Autodesk Inventor part; units mm, degrees
ref_plane "YZ Plane" through (0, 0, 0) normal (1, 0, 0) x (0, 1, 0)
ref_plane "XZ Plane" through (0, 0, 0) normal (0, 1, 0) x (-1, 0, 0)
ref_plane "XY Plane" through (0, 0, 0) normal (0, 0, 1) x (1, 0, 0)
sketch "Sketch1" plane through (0, 0, 0) normal (0, 1, 0) x (-1, 0, 0)
  line L0 (2, -96) -> (-2, -96)
  line L1 (-2, -96) -> (-2, 96)
  line L2 (-2, 96) -> (2, 96)
  line L3 (2, 96) -> (2, -96)
  line L4 (2, -96) -> (-2, 96) construction
  line L5 (-2, -96) -> (2, 96) construction
  circle A0 centre (0, 94) radius 0.85
  circle A1 centre (0, -94) radius 0.85
  circle A2 centre (0, 0) radius 0.85
  circle A3 centre (0, 48) radius 0.85
  circle A4 centre (0, -48) radius 0.85
  point P0 (0, 0)
  dimension "d0" = 192
  dimension "d1" = 4
  dimension "d2" = 1.7
  dimension "d3" = 2
  dimension "d4" = 2
  dimension "d5" = 1.7
  dimension "d6" = 2
  dimension "d7" = 2
  dimension "d8" = 1.7
  dimension "d9" = 96
  dimension "d10" = 2
  dimension "d11" = 1.7
  dimension "d12" = 2
  dimension "d13" = 48
  dimension "d14" = 1.7
  dimension "d15" = 2
  dimension "d16" = 48
extrude "MainBody" add sketch "Sketch1" along normal blind 70
sketch "Sketch2" plane through (0, 70, 0) normal (0, 1, 0) x (1, 0, 0)
  circle A0 centre (0, 0) radius 0.85
extrude "MiddlePole" add sketch "Sketch2" along normal blind 3 and the other way blind 70
sketch "Sketch3" plane through (0, 70, 0) normal (0, 1, 0) x (1, 0, 0)
  circle A0 centre (0, -48) radius 0.85
  point P0 (0, 0)
extrude "MiddleLeftPole" add sketch "Sketch3" along normal blind 3 and the other way blind 70
sketch "Sketch4" plane through (0, 70, 0) normal (0, 1, 0) x (1, 0, 0)
  circle A0 centre (0, -94) radius 0.85
  point P0 (0, 0)
extrude "LeftMostPole" add sketch "Sketch4" along normal blind 3 and the other way blind 70
sketch "Sketch5" plane through (0, 70, 0) normal (0, 1, 0) x (1, 0, 0)
  circle A0 centre (0, 48) radius 0.85
  point P0 (0, 0)
extrude "Extrusion5" add sketch "Sketch5" along normal blind 3 and the other way blind 70
sketch "Sketch6" plane through (0, 70, 0) normal (0, 1, 0) x (1, 0, 0)
  circle A0 centre (0, 94) radius 0.85
  point P0 (0, 0)
extrude "Extrusion6" add sketch "Sketch6" along normal blind 3 and the other way blind 70
properties part number "DindingKargoDepanBelakang"
Design review of the part built by this model. Coordinates are the model's own, in mm. Coordinates: 2 decimals unless noted, no trailing zeros. Loops run counter-clockwise (first coordinate to the right, second up) from the corner with the lowest first, then second, coordinate; pieces in that order, holes last.
Q1. To check wall thickness, follow line 1 (Y direction, x = 0.95, z = 58). State the ranges of the line that lie inside material, in increasing order.
Reported:
line 1: y = 0 to 70
Q2. We need section A-A on x = -0.15. State the section outline as (y, z) points, and give its area (3 significant figures).
Reported:
outline: (0, -96) - (70, -96) - (70, -94.84) - (73, -94.84) - (73, -93.16) - (70, -93.16) - (70, -48.84) - (73, -48.84) - (73, -47.16) - (70, -47.16) - (70, -0.84) - (73, -0.84) - (73, 0.84) - (70, 0.84) - (70, 47.16) - (73, 47.16) - (73, 48.84) - (70, 48.84) - (70, 93.16) - (73, 93.16) - (73, 94.84) - (70, 94.84) - (70, 96) - (0, 96) - close
area: 13,500 mm2
Q3. We need section B-B on z = 76.5. State the section outline as (x, y) points.
Reported:
outline: (-2, 0) - (2, 0) - (2, 70) - (-2, 70) - close
Q4. The part is to be moulded in two halves that separate along Z. For faces 1 (the face through (0, 35, 96)), 2 (the face through (0, 35, -96)), 3 (the face through (0, 0, 1)), 4 (the face through (0, 70, 1)), say which applies: +Z half, -Z half, draft (parallel to the pull), parting line (faces both ways), or undercut.
Reported:
face 1: +Z half
face 2: -Z half
face 3: draft
face 4: undercut
